```python
from build123d import *

# Parameters (mm, degrees)
SKETCH2_R           = 0.05
BOSS_EXTRUDE1_DEPTH = 10
SKETCH2_3_R         = 0.05
BOSS_EXTRUDE2_DEPTH = 8.5


with BuildPart() as part:
    # Sketch1 → Revolve1 (revolve)
    with BuildSketch(Plane.XY, mode=Mode.PRIVATE) as revolve1_sk:
        with BuildLine():
            Line((0, 0), (1, 0))
            Line((1, 0), (1, 2))
            ThreePointArc((1, 2), (0.707106781, 2.707106781), (0, 3))
            Line((0, 3), (0, 0))
        make_face()
    revolve(revolve1_sk.sketch.rotate(Axis((0, 4.374977091, 0), (0, -1, 0)), 90), axis=Axis((0, 4.374977091, 0), (0, -1, 0)))

    # Sketch2 → Boss-Extrude1 (add)
    with BuildSketch(Plane.XZ):
        with Locations(Location((-0.85, 0, 0), (0, 0, 90))):
            Circle(SKETCH2_R)
    extrude(amount=BOSS_EXTRUDE1_DEPTH)

    # Sketch2_3 → Boss-Extrude2 (add)
    with BuildSketch(Plane.XZ):
        with Locations(Location((0.85, 0, 0), (0, 0, 90))):
            Circle(SKETCH2_3_R)
    extrude(amount=BOSS_EXTRUDE2_DEPTH)


solid = part.part
```
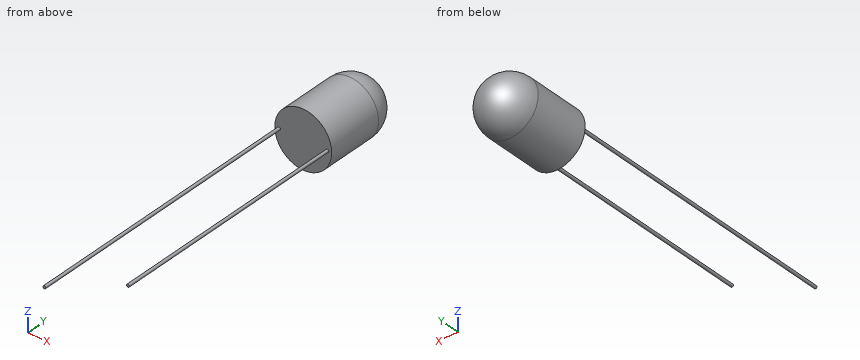
Part model, mm, in its own coordinate system. Round coordinates to 2 decimals unless told otherwise and drop trailing zeros. Write each loop counter-clockwise with the first axis right and the second up, starting at its lowest first coordinate (ties: lowest second). Pieces come first, ordered by that corner, then holes. Notation, with made-up numbers: (63, 49) -> (91, 49) arc R35 ccw to (91, 87) -> close; hole circle Ø2 at (28, -23.75). An arc over 180 degrees is marked (long way). Return JSON: item names as keys, results as strings. Group by question number.
Q1. Saw through at B-B on y = 0.75. Write the cut outline in (x, z), plus the area to 3 significant figures.
Q2. Pin check, flat tips, straight feed: pin 1 (1 mm diameter, centred on x = -0.5, z = 0.5, fed in from -Y); pin 2 (1 mm diameter, centred on x = 1, z = 0, fed in from +Y). Stop position of each tip, or through.
Q3. Saw through at C-C on z = -0.45. Write the cut outline in (x, y).
Q4. Saw through at A-A on x = 0. Write the cut outline in (y, z), plus the area to 3 significant figures.
Q5. Probe L1, parallel to Z at x = 0.05, y = 1.75; L2, parallel to Y at x = 0.45, z = -0.75; L3, parallel to X at y = 2, z = 0.6. List the from-to ranges inside material, lowest first. Write a range as [from, to].
Answer:
{
 "1": {"outline": "circle Ø2 at (0, 0)", "area": "3.14 mm2"},
 "2": {"pin 1": "y = 0", "pin 2": "y = 2.87"},
 "3": {"outline": "(-0.89, 0) -> (0.89, 0) -> (0.89, 2) arc R0.89 ccw to (-0.89, 2) -> close"},
 "4": {"outline": "(0, -1) -> (2, -1) arc R1 ccw to (2, 1) -> (0, 1) -> close", "area": "5.57 mm2"},
 "5": {"L1": "[-1, 1]", "L2": "[0, 2.48]", "L3": "[-0.8, 0.8]"}
}
